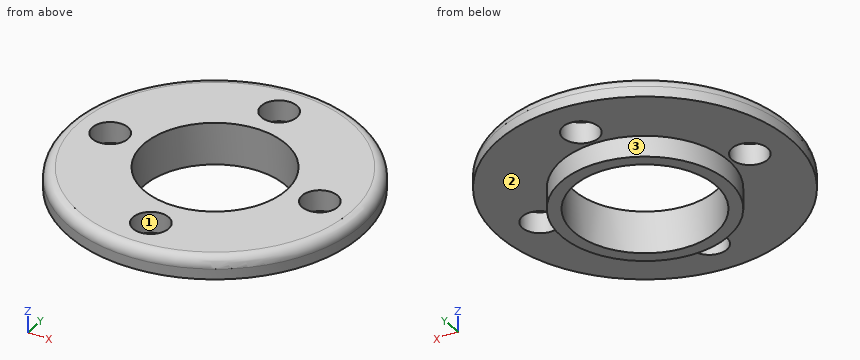
from build123d import *

# Parameters (mm, degrees)
CIRPATTERN1_COUNT = 4
FILLET1_R         = 1


with BuildPart() as part:
    # Sketch1 → Revolve1 (revolve)
    with BuildSketch(Plane(origin=(0, 0, 0), x_dir=(0, 0, -1), z_dir=(1, 0, 0))):
        Polygon((-1, 14), (1, 14), (1, 8), (3, 8), (3, 6.8), (-1, 6.8), align=None)
    revolve(axis=Axis((0, 0, -88.99), (0, 0, 1)))

    # Sketch4 → M3 Clearance Hole1 (revolve, cut)
    with BuildSketch(Plane(origin=(10, 0, 1), x_dir=(0, -1, 0), z_dir=(1, 0, 0))):
        Polygon((0, 0), (0, 9.021463052), (1.7, 8), (1.7, 0), align=None)
    m3_clearance_hole1 = revolve(axis=Axis((10, 0, 7.35), (0, 0, -1)), mode=Mode.SUBTRACT)

    # CirPattern1: M3 Clearance Hole1 ×4 about axis
    cirpattern1_axis = Axis((0, 0, 0), (0, 0, 1))
    for i in range(1, CIRPATTERN1_COUNT):
        add(m3_clearance_hole1.rotate(cirpattern1_axis, i * 360 / CIRPATTERN1_COUNT), mode=Mode.SUBTRACT)

    # Fillet1
    fillet1_edges = [part.edges().sort_by_distance(p)[0] for p in [
        (0, -14, 1),
    ]]
    fillet(fillet1_edges, radius=FILLET1_R)


solid = part.part
Part model, mm, in its own coordinate system. Face numbers are marked on the shaded views. Give positions to 0.01 mm unless a question says otherwise; leave off trailing zeros. Loops run counter-clockwise (first coordinate to the right, second up) from the corner with the lowest first, then second, coordinate; pieces in that order, holes last. Notation, with made-up numbers: (4, 86) -> (17, 86) arc R25 ccw to (17, 119) -> close; hole circle Ø11 at (-35.5, 3.25). An arc over 180 degrees is marked (long way). Write each question's results on one line, items separated by ' | '. Start each with the question number.
Q1. Pull direction Y, two halves, no side cores. Call the marked faces 1, 2 and 3: +Y half, -Y half, draft (parallel to the pull), parting line (faces both ways), or undercut.
Q2. Band-saw the part on A-A on y = 0. List the corners of the cut face in (x, z), plus the area to 3 significant figures.
Q3. Pin check, flat tip, straight feed: P1, Ø1.5, axis at x = -8, z = -0.5, coming from the +Y side. Stop position of the tip, or through.
Q4. Band-saw the part on B-B on z = -1.95. List the corners of the cut face in (x, y), plus the area to 3 significant figures.
Q5. Wall check: L1, parallel to Y at x = 0, z = -0.05; L2, parallel to Z at x = 11.5, y = 4.25. Give the ranges that are in metal, low to high.
Results are:
1) face 1: undercut | face 2: draft | face 3: parting line
2) outline: (-14, -1) -> (-11.7, -1) -> (-11.7, 1) -> (-13, 1) arc R1 ccw to (-14, 0) -> close; (-8.3, -1) -> (-8, -1) -> (-8, -3) -> (-6.8, -3) -> (-6.8, 1) -> (-8.3, 1) -> close; (6.8, -3) -> (8, -3) -> (8, -1) -> (8.3, -1) -> (8.3, 1) -> (6.8, 1) -> close; (11.7, -1) -> (14, -1) -> (14, 0) arc R1 ccw to (13, 1) -> (11.7, 1) -> close | area: 19.6 mm²
3) P1: stops at y = 11.98
4) outline: circle Ø16 at (0, 0); hole circle Ø13.6 at (0, 0) | area: 55.8 mm²
5) L1: y = -14 to -11.7, -8.3 to -6.8, 6.8 to 8.3, 11.7 to 14 | L2: z = -1 to 1
